Check sheet for the modelled part. Datum: model origin and axes. Units: mm. Round coordinates to 2 decimals unless told otherwise and drop trailing zeros. Loops run counter-clockwise (first coordinate to the right, second up) from the corner with the lowest first, then second, coordinate; pieces in that order, holes last. Notation, with made-up numbers: (-29, 87) -> (-18, 87) arc R31 ccw to (-18, 114) -> close; hole circle Ø11 at (22, 43.5). An arc over 180 degrees is marked (long way). Return JSON: item names as keys, results as strings.
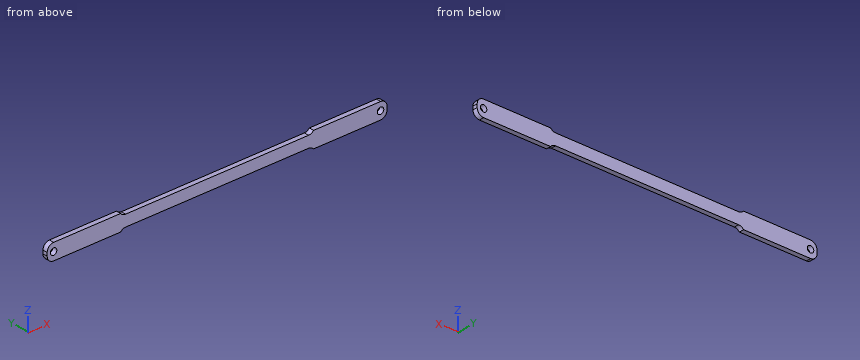
from build123d import *

# Parameters (mm, degrees)
SKETCH2_R           = 1
BOSS_EXTRUDE1_DEPTH = 1.5
SKETCH3_W           = 60
SKETCH3_H           = 1.5
CUT_EXTRUDE1_DEPTH  = 53.900400755
FILLET1_R           = 2


with BuildPart() as part:
    # Sketch2 → Boss-Extrude1 (new body)
    with BuildSketch(Plane(origin=(0, 0, 0), x_dir=(1, 0, 0), z_dir=(0, 1, 0))):
        with BuildLine():
            Line((-50.82, 2.5), (50.82, 2.5))
            ThreePointArc((50.82, 2.5), (52.234213562, 1.914213562), (52.82, 0.5))
            Line((52.82, 0.5), (52.82, -0.5))
            ThreePointArc((52.82, -0.5), (52.234213562, -1.914213562), (50.82, -2.5))
            Line((50.82, -2.5), (-50.82, -2.5))
            ThreePointArc((-50.82, -2.5), (-52.234213562, -1.914213562), (-52.82, -0.5))
            Line((-52.82, -0.5), (-52.82, 0.5))
            ThreePointArc((-52.82, 0.5), (-52.234213562, 1.914213562), (-50.82, 2.5))
        make_face()
        with Locations(Location((-50.82, 0, 0), (0, 0, 270))):
            Circle(SKETCH2_R, mode=Mode.SUBTRACT)
        with Locations(Location((50.82, 0, 0), (0, 0, 270))):
            Circle(SKETCH2_R, mode=Mode.SUBTRACT)
    extrude(amount=BOSS_EXTRUDE1_DEPTH)

    # Sketch3 → Cut-Extrude1 (cut, through all)
    with BuildSketch(Plane(origin=(0, 1.5, 0), x_dir=(1, 0, 0), z_dir=(0, 1, 0))):
        with Locations((0, 2.5)):
            Rectangle(SKETCH3_W, SKETCH3_H)
        with Locations((0, -2.5)):
            Rectangle(SKETCH3_W, SKETCH3_H)
    extrude(amount=-CUT_EXTRUDE1_DEPTH, mode=Mode.SUBTRACT)

    # Fillet1
    # the kernel refuses this fillet: 2 mm, written as the material it adds along each edge
    with BuildSketch(Plane(origin=(30, 1.5, -1.75), x_dir=(0, 0, -1), z_dir=(0, -1, 0)), Plane(origin=(-30, 1.5, 1.75), x_dir=(0, 0, 1), z_dir=(0, -1, 0))) as fillet1_piece_1:
        with BuildLine():
            CenterArc((2, -1.5612495), FILLET1_R, 128.682187453, 51.317812547)
            Line((0, -1.5612495), (-0.04, -1.5612495))
            Line((-0.04, -1.5612495), (-0.04, 0))
            Line((-0.04, 0), (0, 0.04))
            ThreePointArc((0, 0.04), (0.375, 0.04), (0.725, 0.03122499))
            Line((0.725, 0.03122499), (0.75, 0))
        make_face()
    extrude(amount=1.5)
    with BuildSketch(Plane(origin=(30, 1.5, 1.75), x_dir=(-1, 0, 0), z_dir=(0, -1, 0))) as fillet1_piece_2:
        with BuildLine():
            CenterArc((1.5612495, -2), FILLET1_R, 90, 51.317812547)
            Line((0, -0.75), (-0.03122499, -0.725))
            ThreePointArc((-0.03122499, -0.725), (-0.04, -0.375), (-0.04, 0))
            Line((-0.04, 0), (0, 0.04))
            Line((0, 0.04), (1.5612495, 0.04))
            Line((1.5612495, 0.04), (1.5612495, 0))
        make_face()
    extrude(amount=1.5)
    with BuildSketch(Plane(origin=(-30, 1.5, -1.75), x_dir=(0, 0, -1), z_dir=(0, -1, 0))) as fillet1_piece_3:
        with BuildLine():
            CenterArc((2, 1.5612495), FILLET1_R, 180, 51.317812547)
            Line((0, 1.5612495), (-0.04, 1.5612495))
            Line((-0.04, 1.5612495), (-0.04, 0))
            Line((-0.04, 0), (0, -0.04))
            ThreePointArc((0, -0.04), (0.375, -0.04), (0.725, -0.03122499))
            Line((0.725, -0.03122499), (0.75, 0))
        make_face()
    extrude(amount=1.5)


solid = part.part
Q1. Section check A-A (y = 1). Record the boundary of the cut face in (x, z).
Results list:
{"outline": "(-52.82, -0.5) arc R2 ccw to (-50.82, -2.5) -> (-30, -2.5) arc R2 cw to (-28.44, -1.75) -> (28.44, -1.75) arc R2 cw to (30, -2.5) -> (50.82, -2.5) arc R2 ccw to (52.82, -0.5) -> (52.82, 0.5) arc R2 ccw to (50.82, 2.5) -> (30, 2.5) arc R2 cw to (28.44, 1.75) -> (-28.44, 1.75) arc R2 cw to (-30, 2.5) -> (-50.82, 2.5) arc R2 ccw to (-52.82, 0.5) -> close; hole circle Ø2 at (-50.82, 0); hole circle Ø2 at (50.82, 0)"}
Q2. Material ranges on line 1 (X direction, y = 0.95, z = 0); line 2 (Z direction, x = 4, y = 1.1); line 3 (X direction, y = 0.5, z = 2.2), recorded low to high.
Results list:
{"line 1": "-52.82 to -51.82, -49.82 to 49.82, 51.82 to 52.82", "line 2": "-1.75 to 1.75", "line 3": "-51.87 to -29.7, 29.7 to 51.87"}
Q3. Section check B-B (x = -21.5). Record the boundary of the cut face in (y, z).
Results list:
{"outline": "(0, -1.75) -> (1.5, -1.75) -> (1.5, 1.75) -> (0, 1.75) -> close"}
